Source: CAD feature listing. Evaluate the final solid. Frame: model axes, mm. A direction names the side the tool comes from. Give positions to 0.01 mm unless a question says otherwise; leave off trailing zeros. Write each loop counter-clockwise with the first axis right and the second up, starting at its lowest first coordinate (ties: lowest second). Pieces come first, ordered by that corner, then holes. Notation, with made-up numbers: (28, -28.5) -> (46, -28.5) arc R19 cw to (46, -19.5) -> close; hole circle Ø10 at (49.25, 76.5). An arc over 180 degrees is marked (long way). Write item = value, one per line.
from build123d import *

# Parameters (mm, degrees)
SKETCH2_W               = 98.8
SKETCH2_H               = 74.5
BASE_FLANGE1_DEPTH      = 3
KENAR_FLAN_1_DEPTH      = 65
KENAR_FLAN_1_START      = 3
KENAR_FLAN_1_PROFILE_W  = 65
KENAR_FLAN_1_PROFILE_H  = 54.2634
KENAR_FLAN_1_PROFILE_R  = 6.5
KENAR_FLAN_1_FLAT_DEPTH = 3
SKETCH10_R              = 3.25
CUT_EXTRUDE2_DEPTH      = 10


# Sheet-metal steps are written as plain solids
with BuildPart() as part:
    # Sketch2 → Base-Flange1 (new body)
    with BuildSketch(Plane.XY):
        Rectangle(SKETCH2_W, SKETCH2_H)
    extrude(amount=-BASE_FLANGE1_DEPTH)

    # Kenar-Flanş1 bend section (across the edge) → Kenar-Flanş1 (add)
    with BuildSketch(Plane(origin=(-50.1366, 32.5, 0), x_dir=(1, 0, 0), z_dir=(0, -1, 0))):
        with BuildLine():
            Line((-3, 0.7366), (0, 0.7366))
            ThreePointArc((0, 0.7366), (0.215745145, 0.215745145), (0.7366, 0))
            Line((0.7366, 0), (0.7366, -3))
            ThreePointArc((0.7366, -3), (-1.905575199, -1.905575199), (-3, 0.7366))
        make_face()
    extrude(amount=KENAR_FLAN_1_DEPTH)

    # Kenar-Flanş1 profile (on flange) → Kenar-Flanş1 flat (add)
    with BuildSketch(Plane(origin=(-50.1366, 0, 0), x_dir=(0, -1, 0), z_dir=(-1, 0, 0)).offset(KENAR_FLAN_1_START)):
        with Locations((0, 27.8683)):
            Rectangle(KENAR_FLAN_1_PROFILE_W, KENAR_FLAN_1_PROFILE_H)
        with Locations((9.057623393, 24.966787755)):
            Circle(KENAR_FLAN_1_PROFILE_R, mode=Mode.SUBTRACT)
        with Locations((-10.75, 25)):
            Circle(KENAR_FLAN_1_PROFILE_R, mode=Mode.SUBTRACT)
    extrude(amount=-KENAR_FLAN_1_FLAT_DEPTH)

    # Sketch10 → Cut-Extrude2 (cut)
    with BuildSketch(Plane.XY):
        with Locations((40.6634, -26.75)):
            Circle(SKETCH10_R)
        with Locations((-4.3366, -26.75)):
            Circle(SKETCH10_R)
        with Locations((-4.3366, 28.25)):
            Circle(SKETCH10_R)
        with Locations((40.6634, 28.25)):
            Circle(SKETCH10_R)
    extrude(amount=-CUT_EXTRUDE2_DEPTH, mode=Mode.SUBTRACT)


solid = part.part
1) Cut plane C-C (x = -5). Return the cut outline in (y, z).
Computed:
outline = (-37.25, -3) -> (-29.93, -3) -> (-29.93, 0) -> (-37.25, 0) -> close; (-23.57, -3) -> (25.07, -3) -> (25.07, 0) -> (-23.57, 0) -> close; (31.43, -3) -> (37.25, -3) -> (37.25, 0) -> (31.43, 0) -> close
2) Access query for faces 5 (the cylindrical face through (38.084, -28.728, -1.479)), 6 (the flat face through (-49.4, -35, -1)), 7 (the flat face through (-50.137, 0, 28)), 8 (the flat face through (-52, 32.5, 26)). Directions: +Z, -Z, +X, -X, +Y, -Y. A direction counts if a zero-diameter tool reaches every point of the face in a straight line with its end or side. Return the directions, or none.
Computed:
face_5 = +Z, -Z
face_6 = +Z, -Z, -X, -Y
face_7 = +Z, +X, +Y, -Y
face_8 = +Z, -Z, -X, +Y
3) Cut plane A-A (y = 10.75). Return the cut outline in (x, z), then the cut area to 3 significant figures.
Computed:
outline = (-53.14, 0.74) arc R3.74 ccw to (-49.4, -3) -> (49.4, -3) -> (49.4, 0) -> (-49.4, 0) arc R0.74 cw to (-50.14, 0.74) -> (-50.14, 18.5) -> (-53.14, 18.5) -> close; (-53.14, 31.5) -> (-50.14, 31.5) -> (-50.14, 55) -> (-53.14, 55) -> close
area = 431 mm²
4) Contact query for flat-ended pins moving along their axis: pin 1 (1.9 mm diameter, centred on x = -51.5, z = 28.5, fed in from -Y); pin 2 (1 mm diameter, centred on x = -30, y = 12, fed in from +Z); pin 3 (15 mm diameter, centred on y = -9.06, z = 24.97, fed in from +X). Output: stop coordinate, or through.
Computed:
pin_1 = -32.5
pin_2 = 0
pin_3 = -50.14
5) Draft query along Z for faces 1 (the cylindrical face through (-51.658, 7.256, 30.481)), 2 (the cylindrical face through (-5.041, -29.923, -1.479)), 3 (the cylindrical face through (-52.013, 0.455, -1.934)), 4 (the cylindrical face through (-51.66, -3.9, 21.01)). Return one class per face: pulls with the +Z half, pulls with the -Z half, needs draft (parallel to the pull), parting line crosses it, or undercut.
Computed:
face_1 = undercut
face_2 = needs draft
face_3 = pulls with the -Z half
face_4 = undercut
6) Material intervals for L1, parallel to X at y = -26, z = -2; L2, parallel to X at y = -21.5, z = 25.5; L3, parallel to Z at x = -29.5, y = -33, sorted ascending.
Computed:
L1 = -51.94 to -7.5, -1.17 to 37.5, 43.83 to 49.4
L2 = -53.14 to -50.14
L3 = -3 to 0
7) Cut plane D-D (y = 28.25). Return the cut outline in (x, z), then the cut area to 3 significant figures.
Computed:
outline = (-53.14, 0.74) arc R3.74 ccw to (-49.4, -3) -> (-7.59, -3) -> (-7.59, 0) -> (-49.4, 0) arc R0.74 cw to (-50.14, 0.74) -> (-50.14, 55) -> (-53.14, 55) -> close; (-1.09, -3) -> (37.41, -3) -> (37.41, 0) -> (-1.09, 0) -> close; (43.91, -3) -> (49.4, -3) -> (49.4, 0) -> (43.91, 0) -> close
area = 431 mm²
8) Cut plane B-B (z = 30). Return the cut outline in (x, y).
Computed:
outline = (-53.14, -32.5) -> (-50.14, -32.5) -> (-50.14, -13.17) -> (-53.14, -13.17) -> close; (-53.14, -4.94) -> (-50.14, -4.94) -> (-50.14, 6.6) -> (-53.14, 6.6) -> close; (-53.14, 14.9) -> (-50.14, 14.9) -> (-50.14, 32.5) -> (-53.14, 32.5) -> close
